Design review of the part built by this model. Coordinates are the model's own, in mm. Face numbers are marked on the shaded views. A direction names the side the tool comes from. Coordinates: 2 decimals unless noted, no trailing zeros. Order: outer loops, then holes, each group sorted by start corner. A loop starts at its lowest first (then second) coordinate and runs counter-clockwise, first axis right, second up. Notation, with made-up numbers: (18, 66) -> (53, 66) arc R23 ccw to (53, 99) -> close; hole circle Ø4 at (16.25, 81.25). An arc over 180 degrees is marked (long way). Use a Markdown table: item, result. Add a question column.
Q1. The part is to be moulded in two halves that separate along Z. For the marked faces 4, 5 and 6, say which applies: pulls with the +Z half, pulls with the -Z half, needs draft (parallel to the pull), parting line crosses it, or undercut.
Q2. Insertion check: pin 1 (10.5 mm diameter, centred on x = 45, y = -39.5, fed in from +Z); pin 2 (8 mm diameter, centred on y = -26.5, z = 65.5, fed in from -X); pin 3 (15 mm diameter, centred on y = -32, z = 46, fed in from +X). Each pin has a flat end and moves straight along its axis. Give the tip position at first contact, or say it passes through.
Q3. Add section C-C (z = 45). State the section outline as (x, y) points.
Q4. Wall thickness on probe 1 along Z at (x, y) = (-27, -19.5); probe 2 along Y at (x, z) = (0, 57.5); probe 3 along Z at (x, y) = (0, -15.5): over which ranges is each line inside the solid? List them lowest first.
Q5. Machinability: for the marked faces 1, 2 and 3, which of the approach directions +Z, -Z, +X, -X, +Y, -Y give a long, thin tool a straight path to every point of the face, cutting with its end or side? Answer none if there is none.
Q6. Add section B-B (y = -3.5). State the section outline as (x, z) points, then the cut area to 3 significant figures.
Q7. Add section A-A (x = 0). State the section outline as (y, z) points, then the cut area to 3 significant figures.
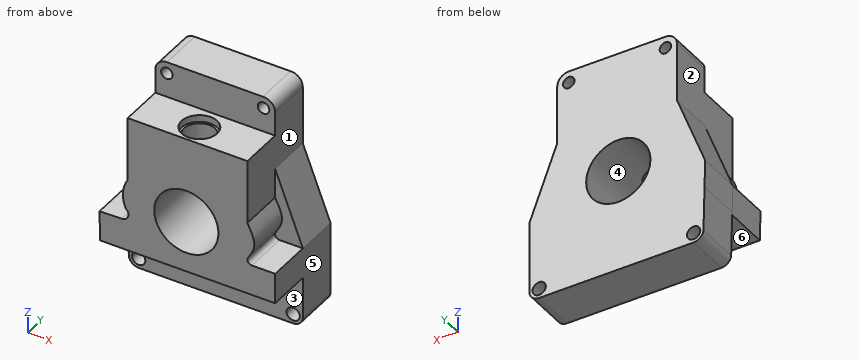
from build123d import *

# Parameters (mm, degrees)
F0_R      = 17.0227145172
F0_R_2    = 3.25
F1_DEPTH  = 25
F2_R      = 3.25
F3_DEPTH  = 70
F4_DEPTH  = 70
F5_R      = 18.1266213474
F6_DEPTH  = 25
F7_DEPTH  = 70
F9_DEPTH  = 25
F5_W      = 67.5716735423
F5_H      = 19.3005736992
F10_DEPTH = 25
F11_R     = 10.0310705793
F12_DEPTH = 3.9
F13_R     = 8.7509220972
F14_DEPTH = 45.3
F15_R     = 3.75
F16_DEPTH = 70
F17_DEPTH = 70


with BuildPart() as f1:
    # F0 (on Front) → F1 (new body)
    with BuildSketch(Plane.XZ):
        with BuildLine():
            Line((34.4588756561, 55.8330058903), (-33.1127978861, 55.8330058903))
            Line((-33.1127978861, 55.8330058903), (-33.1127978861, 40.7908696607))
            Line((-33.1127978861, 40.7908696607), (-33.1127978861, 25.7487334311))
            add(Edge.make_bspline(
                [(-33.1127978861, 25.7487334311), (-34.6033996611, 22.4340609922), (-37.650110278, 15.6590471152), (-34.6467602747, 8.3554726364), (-33.1127978861, 4.625168629)],
                knots=[0, 0, 0, 0, 0.4892495424, 1, 1, 1, 1], degree=3))
            add(Edge.make_bspline(
                [(-33.1127978861, 4.625168629), (-32.7607149389, 2.6646672617), (-32.1126225155, -0.9441018995), (-35.0434349429, -0.2960094761), (-36.3820530474, 0)],
                knots=[0, 0, 0, 0, 0.543260397, 1, 1, 1, 1], degree=3))
            Line((-36.3820530474, 0), (-49.0224920213, -0.2960094761))
            Line((-49.0224920213, -0.2960094761), (-48.661808527, -15.6982113192))
            Line((-48.661808527, -15.6982113192), (50.1245036721, -15.6982113192))
            Line((50.1245036721, -15.6982113192), (50.1245036721, 0))
            Line((50.1245036721, 0), (37.6335456967, 0))
            add(Edge.make_bspline(
                [(34.4588756561, 4.625168629), (34.1095986146, 2.6618613561), (33.4709502093, -0.928019769), (36.3355820401, -0.2893713637), (37.6335456967, 0)],
                knots=[0, 0, 0, 0, 0.5469003581, 1, 1, 1, 1], degree=3))
            add(Edge.make_bspline(
                [(34.4588756561, 25.7487334311), (36.1774809535, 21.1049777281), (39.2730683507, 12.7405489371), (35.9410342162, 7.1236727718), (34.4588756561, 4.625168629)],
                knots=[0, 0, 0, 0, 0.5551790587, 1, 1, 1, 1], degree=3))
            Line((34.4588756561, 25.7487334311), (34.4588756561, 40.7908696607))
            Line((34.4588756561, 40.7908696607), (34.4588756561, 55.8330058903))
        make_face()
        with Locations((0, 12.6643273979)):
            Circle(F0_R, mode=Mode.SUBTRACT)
        with BuildLine():
            Line((50.1245036721, -15.6982113192), (-48.661808527, -15.6982113192))
            Line((-48.661808527, -15.6982113192), (-48.0705925932, -40.9447981115))
            ThreePointArc((-48.0705925932, -40.9447981115), (-46.2339945035, -44.4725848586), (-42.5167828798, -45.8870492876))
            Line((-42.5167828798, -45.8870492876), (44.6597114205, -45.8870492876))
            ThreePointArc((44.6597114205, -45.8870492876), (48.3437920738, -44.4682292272), (50.1245036721, -40.9447981115))
            Line((50.1245036721, -40.9447981115), (50.1245036721, -15.6982113192))
        make_face()
        with Locations((-42.5167828798, -40.2954021766)):
            Circle(F0_R_2, mode=Mode.SUBTRACT)
        with Locations((44.6597114205, -40.3946330681)):
            Circle(F0_R_2, mode=Mode.SUBTRACT)
        with BuildLine():
            ThreePointArc((-26.6140252352, 80.306276679), (-31.2003440388, 78.4118406934), (-33.1127978861, 73.8330058903))
            Line((-33.1127978861, 73.8330058903), (-33.1127978861, 55.8330058903))
            Line((-33.1127978861, 55.8330058903), (34.4588756561, 55.8330058903))
            Line((34.4588756561, 55.8330058903), (34.4588756561, 73.807453795))
            ThreePointArc((34.4588756561, 73.807453795), (32.4062242428, 78.5527695695), (27.542417869, 80.306276679))
            Line((27.542417869, 80.306276679), (-26.6140252352, 80.306276679))
        make_face()
        with Locations((-26.6140252352, 73.807453795)):
            Circle(F0_R_2, mode=Mode.SUBTRACT)
        with Locations((27.9474437952, 73.807453795)):
            Circle(F0_R_2, mode=Mode.SUBTRACT)
        with Locations((0, 12.6643273979)):
            Circle(F0_R)
        with BuildLine():
            Line((-33.1127978861, 25.7487334311), (-33.1127978861, 40.7908696607))
            Line((-33.1127978861, 40.7908696607), (-49.0224920213, -0.2960094761))
            Line((-49.0224920213, -0.2960094761), (-36.3820530474, 0))
            add(Edge.make_bspline(
                [(-33.1127978861, 4.625168629), (-32.7607149389, 2.6646672617), (-32.1126225155, -0.9441018995), (-35.0434349429, -0.2960094761), (-36.3820530474, 0)],
                knots=[0, 0, 0, 0, 0.543260397, 1, 1, 1, 1], degree=3))
            add(Edge.make_bspline(
                [(-33.1127978861, 25.7487334311), (-34.6033996611, 22.4340609922), (-37.650110278, 15.6590471152), (-34.6467602747, 8.3554726364), (-33.1127978861, 4.625168629)],
                knots=[0, 0, 0, 0, 0.4892495424, 1, 1, 1, 1], degree=3))
        make_face()
        with BuildLine():
            Line((50.1245036721, 0), (34.4588756561, 40.7908696607))
            Line((34.4588756561, 40.7908696607), (34.4588756561, 25.7487334311))
            add(Edge.make_bspline(
                [(34.4588756561, 25.7487334311), (36.1774809535, 21.1049777281), (39.2730683507, 12.7405489371), (35.9410342162, 7.1236727718), (34.4588756561, 4.625168629)],
                knots=[0, 0, 0, 0, 0.5551790587, 1, 1, 1, 1], degree=3))
            add(Edge.make_bspline(
                [(34.4588756561, 4.625168629), (34.1095986146, 2.6618613561), (33.4709502093, -0.928019769), (36.3355820401, -0.2893713637), (37.6335456967, 0)],
                knots=[0, 0, 0, 0, 0.5469003581, 1, 1, 1, 1], degree=3))
            Line((37.6335456967, 0), (50.1245036721, 0))
        make_face()
        with Locations((-26.6140252352, 73.807453795)):
            Circle(F0_R_2)
        with Locations((27.9474437952, 73.807453795)):
            Circle(F0_R_2)
        with Locations((-42.5167828798, -40.2954021766)):
            Circle(F0_R_2)
        with Locations((44.6597114205, -40.3946330681)):
            Circle(F0_R_2)
    extrude(amount=F1_DEPTH)

    # F2 (on face) → F3 (cut)
    with BuildSketch(Plane(origin=(0, 0, 0), x_dir=(-1, 0, 0), z_dir=(0, 1, 0))):
        with Locations((-27.9474437952, 73.807453795)):
            Circle(F2_R)
    extrude(amount=-F3_DEPTH, mode=Mode.SUBTRACT)

    # F2 (on face) → F4 (cut)
    with BuildSketch(Plane(origin=(0, 0, 0), x_dir=(-1, 0, 0), z_dir=(0, 1, 0))):
        with Locations((26.6140252352, 73.807453795)):
            Circle(F2_R)
    extrude(amount=-F4_DEPTH, mode=Mode.SUBTRACT)

    # F5 (on face) → F6 (join)
    with BuildSketch(Plane.XZ.offset(25)):
        with BuildLine():
            Line((34.4588756561, 20.5979254097), (34.4588756561, 40.7908696607))
            Line((34.4588756561, 40.7908696607), (-33.1127978861, 40.7908696607))
            Line((-33.1127978861, 40.7908696607), (-33.1127978861, 20.5979254097))
            ThreePointArc((-33.1127978861, 20.5979254097), (-37.1626297585, 12.9749266175), (-34.7937931273, 4.6743325547))
            ThreePointArc((-34.7937931273, 4.6743325547), (-33.9547139722, 1.7822291717), (-36.3820530474, 0))
            Line((-36.3820530474, 0), (-49.0224920213, -0.2960094761))
            Line((-49.0224920213, -0.2960094761), (-48.626471606, -17.2071974467))
            Line((-48.626471606, -17.2071974467), (50.1245036721, -17.2071974467))
            Line((50.1245036721, -17.2071974467), (50.1245036721, 0))
            Line((50.1245036721, 0), (37.3762585223, 0))
            ThreePointArc((37.3762585223, 0), (34.6582437375, 2.1242313939), (36.0628159286, 5.2749678705))
            ThreePointArc((36.0628159286, 5.2749678705), (37.5665970474, 13.1778026111), (34.4588756561, 20.5979254097))
        make_face()
        with Locations((0, 11.75764855)):
            Circle(F5_R, mode=Mode.SUBTRACT)
        with BuildLine():
            Line((-33.1127978861, 20.5979254097), (-33.1127978861, 40.7908696607))
            Line((-33.1127978861, 40.7908696607), (-49.0224920213, -0.2960094761))
            Line((-49.0224920213, -0.2960094761), (-36.3820530474, 0))
            ThreePointArc((-36.3820530474, 0), (-33.9547139722, 1.7822291717), (-34.7937931273, 4.6743325547))
            ThreePointArc((-34.7937931273, 4.6743325547), (-37.1626297585, 12.9749266175), (-33.1127978861, 20.5979254097))
        make_face()
        with BuildLine():
            Line((50.1245036721, 0), (34.4588756561, 40.7908696607))
            Line((34.4588756561, 40.7908696607), (34.4588756561, 20.5979254097))
            ThreePointArc((34.4588756561, 20.5979254097), (37.5665970474, 13.1778026111), (36.0628159286, 5.2749678705))
            ThreePointArc((36.0628159286, 5.2749678705), (34.6582437375, 2.1242313939), (37.3762585223, 0))
            Line((37.3762585223, 0), (50.1245036721, 0))
        make_face()
    extrude(amount=F6_DEPTH)

    # F7 (cut): a face of the model
    f7_faces = [f1.faces().sort_by_distance(p)[0] for p in [
        (0, -25, 11.75764855),
    ]]
    extrude(f7_faces, amount=-F7_DEPTH, mode=Mode.SUBTRACT)

    # F8 (on face) → F9 (cut)
    with BuildSketch(Plane.XZ.offset(50)):
        with BuildLine():
            Line((-33.1127978861, 23.9283517003), (-33.1127978861, 40.7908696607))
            Line((-33.1127978861, 40.7908696607), (-49.0224920213, -0.2960094761))
            Line((-49.0224920213, -0.2960094761), (-36.3820530474, 0))
            ThreePointArc((-36.3820530474, 0), (-32.8674732325, 2.5960168229), (-34.120904149, 6.7817647319))
            ThreePointArc((-34.120904149, 6.7817647319), (-35.7939711067, 15.4830585232), (-33.1127978861, 23.9283517003))
        make_face()
        with BuildLine():
            Line((50.1245036721, 0), (34.4588756561, 40.7908696607))
            Line((34.4588756561, 40.7908696607), (34.4588756561, 23.9283517003))
            add(Edge.make_bspline(
                [(34.4588756561, 23.9283517003), (36.4646656644, 20.023537046), (40.3133082853, 12.5311096019), (36.3544858645, 6.1672411956), (34.4588756561, 3.1200184021)],
                knots=[0, 0, 0, 0, 0.5211681639, 1, 1, 1, 1], degree=3))
            ThreePointArc((34.4588756561, 3.1200184021), (34.9800199126, 0.9572074446), (36.9882769883, 0))
            Line((36.9882769883, 0), (50.1245036721, 0))
        make_face()
    extrude(amount=-F9_DEPTH, mode=Mode.SUBTRACT)

    # F5 (on face) → F10 (join)
    with BuildSketch(Plane.XZ.offset(25)):
        with Locations((0.673038885, 50.4411565103)):
            Rectangle(F5_W, F5_H)
    extrude(amount=F10_DEPTH)

    # F11 (on face) → F12 (cut)
    with BuildSketch(Plane.XY.offset(60.0914433599)):
        with Locations((0, -38.2113941014)):
            Circle(F11_R)
    extrude(amount=-F12_DEPTH, mode=Mode.SUBTRACT)

    # F13 (on face) → F14 (cut)
    with BuildSketch(Plane.XY.offset(56.1914433599)):
        with Locations((0, -38.2113941014)):
            Circle(F13_R)
    extrude(amount=-F14_DEPTH, mode=Mode.SUBTRACT)

    # F15 (on face) → F16 (cut)
    with BuildSketch(Plane.XZ.offset(25)):
        with Locations((-42.5167828798, -40.2954021766)):
            Circle(F15_R)
    extrude(amount=-F16_DEPTH, mode=Mode.SUBTRACT)

    # F15 (on face) → F17 (cut)
    with BuildSketch(Plane.XZ.offset(25)):
        with Locations((44.6597114205, -40.3946330681)):
            Circle(F15_R)
    extrude(amount=-F17_DEPTH, mode=Mode.SUBTRACT)


solid = f1.part
Established:
| question | item | result |
|---|---|---|
| 1 | face 4 | undercut |
| 1 | face 5 | needs draft |
| 1 | face 6 | pulls with the -Z half |
| 2 | pin 1 | z = 0 |
| 2 | pin 2 | x = -33.11 |
| 2 | pin 3 | x = 34.46 |
| 3 | outline | (-33.11, -50) -> (34.46, -50) -> (34.46, 0) -> (-33.11, 0) -> close; hole circle Ø17.5 at (0, -38.21) |
| 4 | probe 1 | -45.89 to 70.58, 77.03 to 80.29 |
| 4 | probe 2 | -50 to -48.24, -28.18 to 0 |
| 4 | probe 3 | -45.89 to -6.37, 29.88 to 80.31 |
| 5 | face 1 | +Z, +X, -Y |
| 5 | face 2 | +Z, -X, -Y |
| 5 | face 3 | -Z, +X, -X, -Y |
| 6 | outline | (-49.02, -0.3) -> (-48.07, -40.94) arc R5.59 ccw to (-42.52, -45.89) -> (44.66, -45.89) arc R5.49 ccw to (50.12, -40.94) -> (50.12, 0) -> (34.46, 40.79) -> (34.46, 73.81) arc R6.51 ccw to (27.54, 80.31) -> (-26.61, 80.31) arc R6.5 ccw to (-33.11, 73.83) -> (-33.11, 40.79) -> close; hole circle Ø7.5 at (-42.52, -40.3); hole circle Ø6.5 at (-26.61, 73.81); hole circle Ø36.25 at (0, 11.76); hole circle Ø6.5 at (27.95, 73.81); hole circle Ø7.5 at (44.66, -40.39) |
| 6 | area | 9,380 mm^2 |
| 7 | outline | (-50, -17.21) -> (-25, -17.21) -> (-25, -45.89) -> (0, -45.89) -> (0, -6.37) -> (-50, -6.37) -> close; (-50, 29.88) -> (-46.96, 29.88) -> (-46.96, 56.19) -> (-48.24, 56.19) -> (-48.24, 60.09) -> (-50, 60.09) -> close; (-29.46, 29.88) -> (0, 29.88) -> (0, 80.31) -> (-25, 80.31) -> (-25, 60.09) -> (-28.18, 60.09) -> (-28.18, 56.19) -> (-29.46, 56.19) -> close |
| 7 | area | 2,740 mm^2 |
